Autodesk Inventor part; units mm, degrees
ref_plane "IDS_WORKPLANE{1}" through (-5.4864, 0, 0) normal (1, 0, 0) x (0, 0, -1)
ref_plane "Work Plane2" through (41.275, 0, 0) normal (0, 0, -1) x (1, 0, 0)
ref_plane "YZ Plane" through (0, 0, 0) normal (1, 0, 0) x (0, 1, 0)
sketch "Sketch1" plane through (0, 0, 0) normal (0, 0, 1) x (1, 0, 0)
  line L0 (-5.4864, 0) -> (12.7, 0)
  line L1 (12.7, 0) -> (12.7, 3.175)
  line L2 (12.7, 3.175) -> (3.175, 3.175)
  line L3 (3.175, 3.175) -> (2.413, 3.175)
  line L4 (2.413, 3.175) -> (0, 3.175)
  line L5 (0, 3.175) -> (0, 4.7625)
  line L6 (-9.4999, 0) -> (16.4, 0)
  line L7 (0, -0.9693) -> (0, 5.8158)
  line L8 (0, 4.7625) -> (-4.2103, 4.7625)
  arc A0 (-4.2103, 4.7625) -> (-5.4864, 0) centre (4.0386, 0) ccw
  line L9 (3.175, 3.175) -> (0, 3.175) construction
  dimension "d0" = 12.7
  dimension "d1" = 9.525
  dimension "d2" = 0.762
  dimension "d3" = 5.4864
  dimension "d4" = 6.35
  dimension "d5" = 6.35
  dimension "d9" = 9.525
  dimension "d10" = 0
  dimension "d13" = 9.525
revolve "Body" add sketch "Sketch1" angle 360 about axis through (-5.4864, 0, 0) along (1, 0, 0)
ref_plane "IDS_WORKPLANE{1}" through (-5.4864, 0, 0) normal (1, 0, 0) x (0, 0, -1)
sketch "Sketch2" plane through (-5.4864, 0, 0) normal (1, 0, 0) x (0, 0, -1)
  circle A0 centre (0, 0) radius 4.7625
  line L0 (0, -6.6675) -> (0, 6.6675)
  line L1 (6.6675, 0) -> (-6.6675, 0)
  line L2 (-4.7625, 0.9525) -> (4.7625, 0.9525)
  line L3 (4.7625, 0.9525) -> (4.7625, -0.9525)
  line L4 (4.7625, -0.9525) -> (-4.7625, -0.9525)
  line L5 (-4.7625, -0.9525) -> (-4.7625, 0.9525)
  line L6 (-4.7625, 0) -> (4.7625, 0) construction
  line L7 (0, 0.9525) -> (0, -0.9525) construction
  dimension "d15" = 1.905
extrude "Slot" cut sketch "Sketch2" along normal blind 2.4638 contours L1 L0 L2 A0 | L3 L4 A0 | A0 L4 L0 L1 | A0 L2 L3 | L1 A0 L2 L0 | L0 L4 A0 L1 | L5 L2 A0 | A0 L4 L5
thread "Thread"
sketch "Sketch3" plane through (0, 0, 0) normal (0, 0, 1) x (1, 0, 0)
  line L0 (12.7, 0) -> (12.7, 3.175)
  line L1 (12.7, 3.175) -> (3.175, 3.175)
  line L2 (-5.4864, 0) -> (12.7, 0)
  arc A0 (12.7, 0) -> (11.8493, 3.175) centre (6.35, 0) ccw
  line L3 (12.7, -3.175) -> (12.7, 3.175)
  line L4 (11.8493, 3.175) -> (11.8493, 0)
  line L5 (11.8493, 0) -> (12.7, 0)
  dimension "d40" = 6.35
revolve "Fillet1" cut sketch "Sketch3" angle 360 about axis through (-5.4864, 0, 0) along (1, 0, 0) contours A0 L1 L0
chamfer "Chamfer" distance 0.635 angle 45 1 edges at (11.8493, -3.175, 0)
ref_plane "Work Plane2" through (41.275, 0, 0) normal (0, 0, -1) x (1, 0, 0)
fillet "Fillet4" radius 0.7874 1 edges at (0, -3.175, 0)
equation "\"d0\" = NLG"
equation "\"d1\" = GEL"
equation "\"d2\" = GAL"
equation "\"d3\" = KOH"
equation "\"d4\" = GD"
equation "\"d5\" = BDM"
equation "\"d9\" = KOD"
equation "\"d13\" = KR"
equation "\"d15\" = SBR"
equation "\"d16\" = STI"
equation "\"d40\" = GD"
equation "\"d46\" = R"
equation "\"d11\" = GEL"
equation "\"d43\" = 0.5 * RR"
equation "\"GD\" = NND"
equation "\"NLG\" = 12.7"
equation "\"GEL\" = 9.525"
equation "\"KOD\" = 9.525"
equation "\"KOH\" = 5.4864"
equation "\"GAL\" = 0.762"
equation "\"BDM\" = NND"
equation "\"SBR\" = 1.905"
equation "\"STI\" = 2.4638"
equation "\"KEWI\" = 0"
equation "\"KR\" = KOD"
equation "\"d14\" = -KOH"
equation "\"R\" = 0.7874"
equation "\"THREADDIA\" = 6.35"
equation "\"TOA\" = 30deg"
equation "\"KOH1\" = 4.3688"
equation "\"NND\" = 6.35"
equation "\"GD1\" = 4.8387"
equation "\"THREADDESC\" = 1.2345"
properties part number "ANSI B18.6.2 - 1/4-20 UNC - 0.5, SFHCSI" material "Steel, Mild"
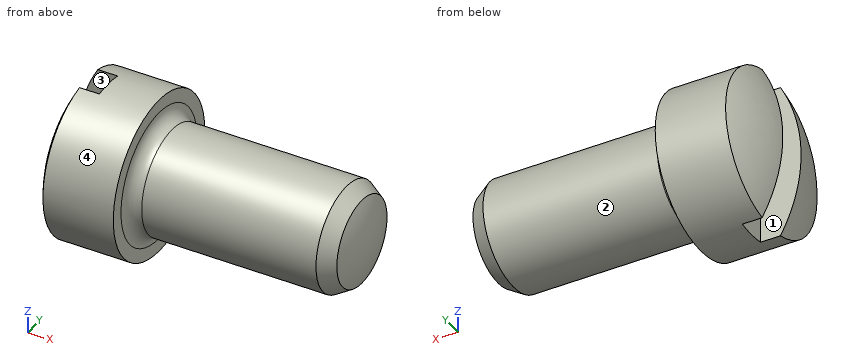
Part model, mm, in its own coordinate system. Face numbers are marked on the shaded views. A direction names the side the tool comes from. Give positions to 0.01 mm unless a question says otherwise; leave off trailing zeros. Loops run counter-clockwise (first coordinate to the right, second up) from the corner with the lowest first, then second, coordinate; pieces in that order, holes last. Notation, with made-up numbers: M 61,33.5 L 101,33.5 A18 cw 101,68.5 Z; hole C 53.5,-1.5 d3. An arc over 180 degrees is marked long. Put each result on its own line as item: value. Start each with the question number.
1) 3-axis set-ups, long thin cutter, end or side, ignore diameter. For the marked faces 3 and 4: which of +Z, -Z, +X, -X, +Y, -Y reach the whole face in a straight line?
2) Saw through at B-B (x = -0.5). List the corners of the cut face in (y, z) (1 decimal).
3) Pull direction Y, two halves, no side cores. Call the marked faces 1 and 2: +Y half, -Y half, draft (parallel to the pull), parting line (faces both ways), or undercut.
4) Probe probe 1 along Y at (x, z) = (-4, -2.25); probe 2 along Y at (x, z) = (-3.75, -4); probe 3 along Z at (x, y) = (2.5, 2.5). List the from-to ranges inside material, lowest first.
5) Saw through at A-A (x = 10). List the corners of the cut face in (y, z) (3 decimals), then the cut area to 3 significant figures.
6) Flat gauge pins, fed straight in: pin 1 (1 mm diameter, centred on x = -0.5, y = 1.5, fed in from -Z); pin 2 (1.5 mm diameter, centred on x = -1.5, z = 3.5, fed in from -Y); pin 3 (2 mm diameter, centred on x = 0, y = -2.5, fed in from -Z). Where does each tip first touch, or does it go through?
Numbers:
1. face 3: +Z, -Z, -X
1. face 4: +X, -X
2. outline: C 0,0 d9.5
3. face 1: undercut
3. face 2: parting line
4. probe 1: -4.2 to -0.95, 0.95 to 4.2
4. probe 2: -2.58 to -0.95, 0.95 to 2.58
4. probe 3: -1.96 to 1.96
5. outline: C 0,0 d6.35
5. area: 31.7 mm^2
6. pin 1: z = -4.66
6. pin 2: y = -3.89
6. pin 3: z = -4.52
